from build123d import *

# Parameters (mm, degrees)
BOSS_EXTRUDE1_DEPTH = 50
SKETCH2_R           = 10
BOSS_EXTRUDE3_DEPTH = 6
BOSS_EXTRUDE4_START = -50
SKETCH2_2_R         = 10
BOSS_EXTRUDE4_DEPTH = 50


with BuildPart() as part:
    # Sketch1 → Boss-Extrude1 (new body)
    with BuildSketch(Plane.XY):
        with BuildLine():
            ThreePointArc((3, 49.909918854), (0, 50), (-3, 49.909918854))
            Line((-3, 49.909918854), (-3, 7.242640687))
            Line((-3, 7.242640687), (-33.170321726, 37.412962414))
            ThreePointArc((-33.170321726, 37.412962414), (-35.355339059, 35.355339059), (-37.412962414, 33.170321726))
            Line((-37.412962414, 33.170321726), (-7.242640687, 3))
            Line((-7.242640687, 3), (-49.909918854, 3))
            ThreePointArc((-49.909918854, 3), (-50, 0), (-49.909918854, -3))
            Line((-49.909918854, -3), (-7.242640687, -3))
            Line((-7.242640687, -3), (-37.412962414, -33.170321726))
            ThreePointArc((-37.412962414, -33.170321726), (-35.355339059, -35.355339059), (-33.170321726, -37.412962414))
            Line((-33.170321726, -37.412962414), (-3, -7.242640687))
            Line((-3, -7.242640687), (-3, -49.909918854))
            ThreePointArc((-3, -49.909918854), (0, -50), (3, -49.909918854))
            Line((3, -49.909918854), (3, -7.242640687))
            Line((3, -7.242640687), (33.170321726, -37.412962414))
            ThreePointArc((33.170321726, -37.412962414), (35.355339059, -35.355339059), (37.412962414, -33.170321726))
            Line((37.412962414, -33.170321726), (7.242640687, -3))
            Line((7.242640687, -3), (49.909918854, -3))
            ThreePointArc((49.909918854, -3), (49.97747464, -1.500676065), (50, 0))
            ThreePointArc((50, 0), (49.97747464, 1.500676065), (49.909918854, 3))
            Line((49.909918854, 3), (7.242640687, 3))
            Line((7.242640687, 3), (37.412962414, 33.170321726))
            ThreePointArc((37.412962414, 33.170321726), (35.355339059, 35.355339059), (33.170321726, 37.412962414))
            Line((33.170321726, 37.412962414), (3, 7.242640687))
            Line((3, 7.242640687), (3, 49.909918854))
        make_face()
    extrude(amount=BOSS_EXTRUDE1_DEPTH)

    # Sketch2 → Boss-Extrude3 (add)
    with BuildSketch(Plane.XY.offset(50)):
        with Locations(Location((0, 0, 0), (0, 0, 197.457603124))):
            Circle(SKETCH2_R)
    extrude(amount=BOSS_EXTRUDE3_DEPTH)

    # Sketch2_2 → Boss-Extrude4 (add)
    with BuildSketch(Plane.XY.offset(50).offset(BOSS_EXTRUDE4_START)):
        with Locations(Location((0, 0, 0), (0, 0, 197.457603124))):
            Circle(SKETCH2_2_R)
    extrude(amount=BOSS_EXTRUDE4_DEPTH)


solid = part.part
The listing builds one solid part. Answer for the finished solid, in the listing's coordinates (mm). A direction names the side the tool comes from. Coordinates: 2 decimals unless noted, no trailing zeros. Loops run counter-clockwise (first coordinate to the right, second up) from the corner with the lowest first, then second, coordinate; pieces in that order, holes last. Notation, with made-up numbers: (21, -0.75) -> (31, -0.75) arc R31 ccw to (31, 28.25) -> close; hole circle Ø11 at (20.25, -37). An arc over 180 degrees is marked (long way). Write item = value, one per line. Start each with the question number.
1) Straight lines are drawn through the part: line 1 (Y direction, x = 10.5, z = 22); line 2 (X direction, y = -9, z = 6); line 3 (X direction, y = -23, z = 31). For each, find the intervals that lie inside material, in ascending order. Write a range as from..to.
2) A tool of negligible diameter and unlimited length cuts with its end or side. For faces 1 (the face through (-3, -29, 25)), 2 (the face through (3, 29, 25)), 3 (the face through (4.48, -8.94, 36.17)), 4 (the face through (22.94, 18.7, 24.65)), from which of +Z, -Z, +X, -X, +Y, -Y can it reach the whole face along a straight path? Write none if from no direction.
3) The mould has two halves that part along Y. Classify faces 5 (the face through (-22.94, -18.7, 24.65)), 6 (the face through (0, -29, 50)), 7 (the face through (35.385, 35.326, 24.65)), 8 (the face through (29, -3, 25)): released by +Y, released by -Y, zero draft, split by the parting line, or undercut.
4) A cutting plane is placed at B-B (y = 36). Give the vertices of the cut face in (x, z).
5) A cutting plane is placed at C-C (x = 0). Give the vertices of the cut face in (y, z).
6) A cutting plane is placed at D-D (x = -21). Give the vertices of the cut face in (y, z), then the cut area to 3 significant figures.
7) Given pin 1 Ø10 at (x, y) = (16.5, 15) entering from +Z; pin 2 Ø4 at (x, z) = (34.5, 8) entering from +Y; pin 3 Ø8 at (x, y) = (36, 25) entering from +Z; pin 4 Ø1 at (y, z) = (15, 19.5) entering from -X, each flat-ended and moving along its own axis, determine where each tip first touches the part or whether it passes through.
Responses:
q1.line_1 = -14.74..-6.26, -3..3, 6.26..14.74
q1.line_2 = -13.24..-4.76, -4.36..4.36, 4.76..13.24
q1.line_3 = -27.24..-18.76, -3..3, 18.76..27.24
q2.face_1 = +Z, -Z, -Y
q2.face_2 = +Z, -Z, +Y
q2.face_3 = +Z
q2.face_4 = +Z, -Z, +X
q3.face_5 = undercut
q3.face_6 = zero draft
q3.face_7 = released by +Y
q3.face_8 = undercut
q4.outline = (-34.7, 0) -> (-31.76, 0) -> (-31.76, 50) -> (-34.7, 50) -> close; (-3, 0) -> (3, 0) -> (3, 50) -> (-3, 50) -> close; (31.76, 0) -> (34.7, 0) -> (34.7, 50) -> (31.76, 50) -> close
q5.outline = (-50, 0) -> (50, 0) -> (50, 50) -> (10, 50) -> (10, 56) -> (-10, 56) -> (-10, 50) -> (-50, 50) -> close
q6.outline = (-25.24, 0) -> (-16.76, 0) -> (-16.76, 50) -> (-25.24, 50) -> close; (-3, 0) -> (3, 0) -> (3, 50) -> (-3, 50) -> close; (16.76, 0) -> (25.24, 0) -> (25.24, 50) -> (16.76, 50) -> close
q6.area = 1,150 mm²
q7.pin_1 = 50
q7.pin_2 = 37.41
q7.pin_3 = through
q7.pin_4 = -19.74
